The drawing under review shows one solid part. Ordinate dimensions are in mm from its lowest x, y, z. Round coordinates to 2 decimals unless told otherwise and drop trailing zeros. Loops run counter-clockwise (first coordinate to the right, second up) from the corner with the lowest first, then second, coordinate; pieces in that order, holes last. Notation, with made-up numbers: (-5, 13.5) - (43, 13.5) arc R22 ccw to (43, 27.5) - close; hole circle Ø10 at (-33, 23.5). An arc over 180 degrees is marked (long way). Answer as CSV lines item,"result".
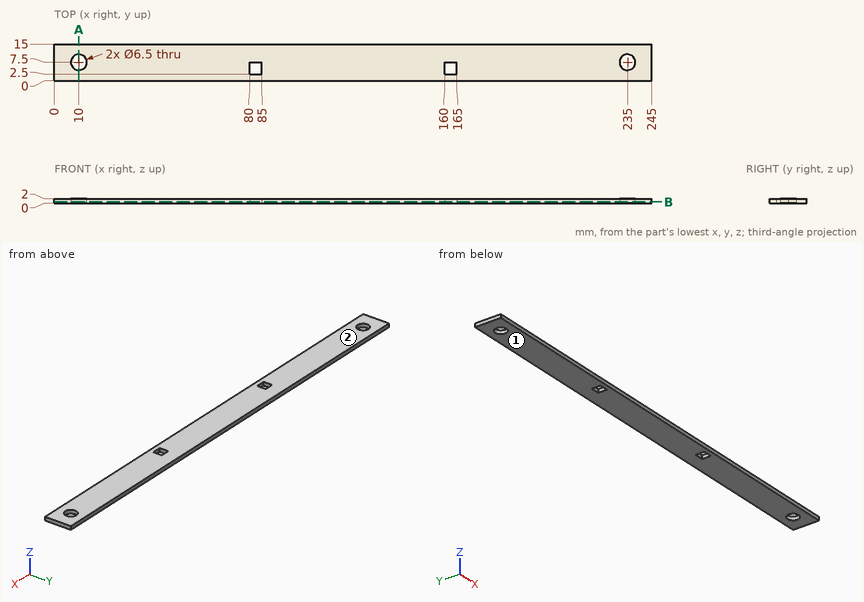
1. Clearance check with a flat-ended pin moving along its axis: pin 1 (1 mm diameter, centred on y = 4.5, z = 1, fed in from -X). State where the tip first meets the part, or that it passes through.
Numbers:
pin 1,"stops at x = 0"
2. Draft analysis for pull direction Z (two halves, no side actions). For the marked faces 1 and 2, state which applies: +Z half, -Z half, draft (parallel to the pull), parting line (faces both ways), or undercut.
Numbers:
face 1,"-Z half"
face 2,"+Z half"
3. Take a section at A-A (x = 10). State the section outline as (y, z) points, plus the area to 3 significant figures.
Numbers:
outline,"(0, 0) - (4.25, 0) - (4.25, 2) - (0, 2) - close; (10.75, 0) - (15, 0) - (15, 2) - (10.75, 2) - close"
area,"17.0 mm²"
4. Take a section at B-B (z = 0.6). State the section outline as (x, y) points.
Numbers:
outline,"(0, 0) - (245, 0) - (245, 15) - (0, 15) - close; hole circle Ø6.5 at (10, 7.5); hole (80, 2.5) - (85, 2.5) - (85, 7.5) - (80, 7.5) - close; hole (160, 2.5) - (165, 2.5) - (165, 7.5) - (160, 7.5) - close; hole circle Ø6.5 at (235, 7.5)"
5. Wall thickness on probe 1 along X at (y, z) = (7, 0.3); probe 2 along Y at (x, z) = (164, 1.1); probe 3 along X at (y, z) = (10, 1.2): over which ranges is each line inside the solid? List them lowest first.
Numbers:
probe 1,"x = 0 to 6.79, 13.21 to 80, 85 to 160, 165 to 231.79, 238.21 to 245"
probe 2,"y = 0 to 2.5, 7.5 to 15"
probe 3,"x = 0 to 7.92, 12.08 to 232.92, 237.08 to 245"
